```python
from build123d import *

# Parameters (mm, degrees)
F1_DEPTH = 12.7


with BuildPart() as f1:
    # F0 (on Front) → F1 (new body)
    with BuildSketch(Plane.XZ):
        Polygon((0, 8.5898101), (0, 0), (135.4050932787, 135.4050932787), (131.1101882287, 139.6999983287), align=None)
        Polygon((135.4050932787, 135.4050932787), (0, 0), (0, -8.5898101), (8.5898101, 0), (139.6999983287, 131.1101882287), align=None)
        Polygon((131.1101882287, 139.6999983287), (135.4050932787, 135.4050932787), (139.6999983287, 139.6999983287), (135.4050932787, 143.9949033787), align=None)
        Polygon((139.6999983287, 139.6999983287), (135.4050932787, 135.4050932787), (139.6999983287, 131.1101882287), (143.9949033787, 135.4050932787), align=None)
        Polygon((0, 270.8101865575), (131.1101882287, 139.6999983287), (135.4050932787, 143.9949033787), (0, 279.3999966575), align=None)
        Polygon((143.9949033787, 143.9949033787), (139.6999983287, 139.6999983287), (143.9949033787, 135.4050932787), (148.2898084287, 139.6999983287), align=None)
        Polygon((135.4050932787, 143.9949033787), (139.6999983287, 139.6999983287), (143.9949033787, 143.9949033787), (139.6999983287, 148.2898084287), align=None)
        Polygon((143.9949033787, 135.4050932787), (139.6999983287, 131.1101882287), (270.8101865575, 0), (279.3999966575, -8.5898101), (279.3999966575, 0), align=None)
        Polygon((0, 279.3999966575), (135.4050932787, 143.9949033787), (139.6999983287, 148.2898084287), (4.29490505, 283.6949017075), (0, 287.9898067575), align=None)
        Polygon((148.2898084287, 139.6999983287), (143.9949033787, 135.4050932787), (279.3999966575, 0), (279.3999966575, 8.5898101), align=None)
        Polygon((139.6999983287, 148.2898084287), (143.9949033787, 143.9949033787), (279.3999966575, 279.3999966575), (279.3999966575, 287.9898067575), (275.1050916075, 283.6949017075), align=None)
        Polygon((279.3999966575, 279.3999966575), (143.9949033787, 143.9949033787), (148.2898084287, 139.6999983287), (279.3999966575, 270.8101865575), align=None)
    extrude(amount=F1_DEPTH)


solid = f1.part
```
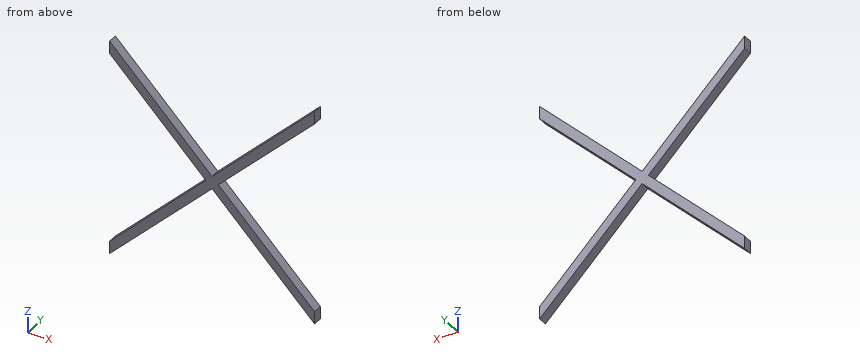
The model under review builds one solid part; all positions refer to its coordinate system, in mm. Round coordinates to 2 decimals unless told otherwise and drop trailing zeros. Order: outer loops, then holes, each group sorted by start corner. A loop starts at its lowest first (then second) coordinate and runs counter-clockwise, first axis right, second up. Notation, with made-up numbers: (29.25, 70) - (63.25, 70) arc R29 ccw to (63.25, 90) - close; hole circle Ø3 at (55.25, 66.5). An arc over 180 degrees is marked (long way). Answer in a Markdown table with one row per item.
(1) For line 1 (X direction, y = -3.5, z = 107.5); line 2 (X direction, y = -5.25, z = 233); line 3 (Z direction, x = 93.5, y = -10.5), list the stretches that pass through material, from the lowest coordinate up. Write a range as from..to.
Result set:
| item | result |
|---|---|
| line 1 | x = 98.91..116.09, 163.31..180.49 |
| line 2 | x = 37.81..54.99, 224.41..241.59 |
| line 3 | z = 84.91..102.09, 177.31..194.49 |
(2) Clearance check with flat-ended pins moving along their axes: P1, Ø2, axis at y = -10, z = 41.5, coming from the +X side; P2, Ø1.5, axis at x = 93, y = -7, coming from the +Z side; P3, Ø4, axis at y = -6, z = 87.5, coming from the +X side. State where each tip first meets the part, or that it passes through.
Result set:
| item | result |
|---|---|
| P1 | stops at x = 247.49 |
| P2 | stops at z = 195.74 |
| P3 | stops at x = 202.49 |
(3) Take a section at A-A on z = 28.5. Write out the cut boundary in (x, y).
Result set:
| item | result |
|---|---|
| outline | (19.91, -12.7) - (37.09, -12.7) - (37.09, 0) - (19.91, 0) - close; (242.31, -12.7) - (259.49, -12.7) - (259.49, 0) - (242.31, 0) - close |
(4) Take a section at C-C on y = -9.5. Write out the cut boundary in (x, z).
Result set:
| item | result |
|---|---|
| outline | (0, -8.59) - (139.7, 131.11) - (279.4, -8.59) - (279.4, 8.59) - (148.29, 139.7) - (279.4, 270.81) - (279.4, 287.99) - (139.7, 148.29) - (0, 287.99) - (0, 270.81) - (131.11, 139.7) - (0, 8.59) - close |
(5) Take a section at D-D on x = 145. Write out the cut boundary in (y, z).
Result set:
| item | result |
|---|---|
| outline | (-12.7, 125.81) - (0, 125.81) - (0, 153.59) - (-12.7, 153.59) - close |
(6) Take a section at B-B on x = 251.5. Write out the cut boundary in (y, z).
Result set:
| item | result |
|---|---|
| outline | (-12.7, 19.31) - (0, 19.31) - (0, 36.49) - (-12.7, 36.49) - close; (-12.7, 242.91) - (0, 242.91) - (0, 260.09) - (-12.7, 260.09) - close |
